```python
from build123d import *

# Parameters (mm, degrees)
F0_W     = 127
F0_H     = 50.8
F1_DEPTH = 25.4
F2_R     = 12.7
F3_DEPTH = 25.4
F4_W     = 236.584601
F4_H     = 130.351219
F4_W_2   = 209.021354
F4_H_2   = 105.084905
F5_DEPTH = 6.35


with BuildPart() as f1:
    # F0 (on Top) → F1 (new body)
    with BuildSketch(Plane.XY):
        Polygon((0, 50.8), (0, 0), (254, 0), (254, 152.4), (0, 152.4), (0, 101.6), align=None)
        with Locations((-63.5, 76.2)):
            Rectangle(F0_W, F0_H)
    extrude(amount=F1_DEPTH)

    # F2 (on face) → F3 (cut)
    with BuildSketch(Plane.XY.offset(25.4)):
        with Locations((-101.6, 76.2)):
            Circle(F2_R)
    extrude(amount=-F3_DEPTH, mode=Mode.SUBTRACT)

    # F4 (on face) → F5 (cut)
    with BuildSketch(Plane.XY.offset(25.4)):
        with Locations((127.957823, 74.994562)):
            Rectangle(F4_W, F4_H)
        with Locations((127.670708, 74.133212)):
            Rectangle(F4_W_2, F4_H_2, mode=Mode.SUBTRACT)
    extrude(amount=-F5_DEPTH, mode=Mode.SUBTRACT)


solid = f1.part
```
Here's how the part is built. I have some questions about the finished solid (model axes, mm). A direction names the side the tool comes from. Coordinates: 2 decimals unless noted, no trailing zeros. Order: outer loops, then holes, each group sorted by start corner. A loop starts at its lowest first (then second) coordinate and runs counter-clockwise, first axis right, second up. Notation, with made-up numbers: M -4.75,24.5 L 16.25,24.5 A13 ccw 16.25,42.5 Z; hole C -8.75,21 d9. An arc over 180 degrees is marked long. Answer as a JSON object with one key per item and string values. Group by question number.
(1) Suppose I cut it at B-B, the plane x = -101.6. Please give me the cut outline in (y, z).
(2) Suppose I cut it at C-C, the plane z = 14.75. Please give me the cut outline in (x, y).
(3) For pin 1 (10 mm diameter, centred on x = -82.5, z = 9.5, fed in from -Y); pin 2 (7 mm diameter, centred on x = 77, z = 22, fed in from -Y); pin 3 (8 mm diameter, centred on y = 36, z = 18.5, fed in from -X), each with a flat end and sliding along its axis, tell me the tip position at first contact or that it passes through.
(4) Which directions (+Z, -Z, +X, -X, +Y, -Y) give clear straight access to the entire face, cutting with the end or side of a thin tool? Please do faces 1 (the face through (-64, 50.8, 13)), 2 (the face through (254, 75, 13)), 3 (the face through (126, 9.819, 22)).
(5) I need wall thicknesses on probe 1 along Y at (x, z) = (28.5, 23.5); probe 2 along X at (y, z) = (113, 21.5); probe 3 along X at (y, z) = (21.5, 23.75). Which ranges of each line are inside material? Lowest first, please.
(6) Suppose I cut it at D-D, the plane y = 27.5. Please give me the cut outline in (x, z), then the cut area to 3 significant figures.
(7) Suppose I cut it at A-A, the plane y = 76.2. Please give me the cut outline in (x, z).
(8) If we mould it in two halves opening along Y, with no side actions, what happens to faces 4 (the face through (-64, 101.6, 13)), 5 (the face through (0, 127, 13)), 6 (the face through (126, 126.676, 22)), 7 (the face through (9.666, 74, 22))? For each: released by +Y, released by -Y, zero draft, split by the parting line, or undercut.
Values found:
{
 "1": {"outline": "M 50.8,0 L 63.5,0 L 63.5,25.4 L 50.8,25.4 Z; M 88.9,0 L 101.6,0 L 101.6,25.4 L 88.9,25.4 Z"},
 "2": {"outline": "M -127,50.8 L 0,50.8 L 0,0 L 254,0 L 254,152.4 L 0,152.4 L 0,101.6 L -127,101.6 Z; hole C -101.6,76.2 d25.4"},
 "3": {"pin 1": "stops at y = 50.8", "pin 2": "stops at y = 0", "pin 3": "stops at x = 0"},
 "4": {"face 1": "+Z, -Z, -X, -Y", "face 2": "+Z, -Z, +X, +Y, -Y", "face 3": "+Z"},
 "5": {"probe 1": "y = 0 to 9.82, 21.59 to 126.68, 140.17 to 152.4", "probe 2": "x = 0 to 9.67, 23.16 to 232.18, 246.25 to 254", "probe 3": "x = 0 to 9.67, 246.25 to 254"},
 "6": {"outline": "M 0,0 L 254,0 L 254,25.4 L 246.25,25.4 L 246.25,19.05 L 232.18,19.05 L 232.18,25.4 L 23.16,25.4 L 23.16,19.05 L 9.67,19.05 L 9.67,25.4 L 0,25.4 Z", "area": "6,280 mm^2"},
 "7": {"outline": "M -127,0 L -114.3,0 L -114.3,25.4 L -127,25.4 Z; M -88.9,0 L 254,0 L 254,25.4 L 246.25,25.4 L 246.25,19.05 L 232.18,19.05 L 232.18,25.4 L 23.16,25.4 L 23.16,19.05 L 9.67,19.05 L 9.67,25.4 L -88.9,25.4 Z"},
 "8": {"face 4": "released by +Y", "face 5": "zero draft", "face 6": "undercut", "face 7": "undercut"}
}
